CAD build for the part. Positions are in the model's coordinates, mm. Face numbers are marked on the shaded views. A direction names the side the tool comes from. Round coordinates to 2 decimals unless told otherwise and drop trailing zeros. Loops run counter-clockwise (first coordinate to the right, second up) from the corner with the lowest first, then second, coordinate; pieces in that order, holes last. Notation, with made-up numbers: M 25.5,88 L 35.5,88 A17 cw 35.5,92 Z; hole C -39,86.25 d1. An arc over 180 degrees is marked long. Use one line per item in the form item = value.
from build123d import *

# Parameters (mm, degrees)
F0_W        = 88.9
F0_H        = 38.1
F1_DEPTH    = 9.144
F2_R        = 4.572
F3_DEPTH    = 12.7
F4_R        = 9.525
F5_DEPTH    = 21.845
F6_SIZE     = 9.144
F7_W        = 9.144
F7_H        = 19.812
F8_DEPTH    = 50.8
F9_T1_DEPTH = 35.2722991577
F10_R       = 4.7625
F11_DEPTH   = 9.144


# Not quite as in the source:
# - a fillet or chamfer that OpenCascade refuses, or shapes differently, is made with other operations: its cross-section is extruded or revolved along the edge and cut away or added


with BuildPart() as f1:
    # F0 (on Front) → F1 (new body)
    with BuildSketch(Plane.XZ):
        with Locations((44.45, 19.05)):
            Rectangle(F0_W, F0_H)
    extrude(amount=F1_DEPTH)

    # F2 (on face) → F3 (join)
    with BuildSketch(Plane.XZ.offset(9.144)):
        with Locations((12.2043658048, 19.05)):
            Circle(F2_R)
    extrude(amount=F3_DEPTH)

    # F4 (on face) → F5 (cut, through all)
    with BuildSketch(Plane(origin=(0, 0, 0), x_dir=(-1, 0, 0), z_dir=(0, 1, 0))):
        with Locations((-76.2, 19.05)):
            Circle(F4_R)
    extrude(amount=-F5_DEPTH, mode=Mode.SUBTRACT)

    # F6
    f6_edges = [f1.edges().sort_by_distance(p)[0] for p in [
        (0, -4.572, 38.1),
        (88.9, -4.572, 38.1),
        (0, -4.572, 0),
        (88.9, -4.572, 0),
    ]]
    chamfer(f6_edges, length=F6_SIZE)

    # F7 (on face) → F8 (join)
    with BuildSketch(Plane.YZ.offset(88.9)):
        with Locations((-4.572, 19.05)):
            Rectangle(F7_W, F7_H)
    extrude(amount=F8_DEPTH)

    # F9: chamfer of 5.08 on 4 edges, made by hand

    # F9_s2 → F9_t1 (cut)
    with BuildSketch(Plane.XZ.offset(-13.0641495789)):
        Polygon((134.62, 28.956), (139.7, 23.876), (139.7, 28.956), align=None)
        Polygon((134.62, 9.144), (139.7, 14.224), (139.7, 9.144), align=None)
    extrude(amount=F9_T1_DEPTH, mode=Mode.SUBTRACT)

    # F10 (on face) → F11 (join)
    with BuildSketch(Plane.XZ.offset(9.144)):
        with Locations((130.556, 18.669)):
            Circle(F10_R)
    extrude(amount=F11_DEPTH)


solid = f1.part
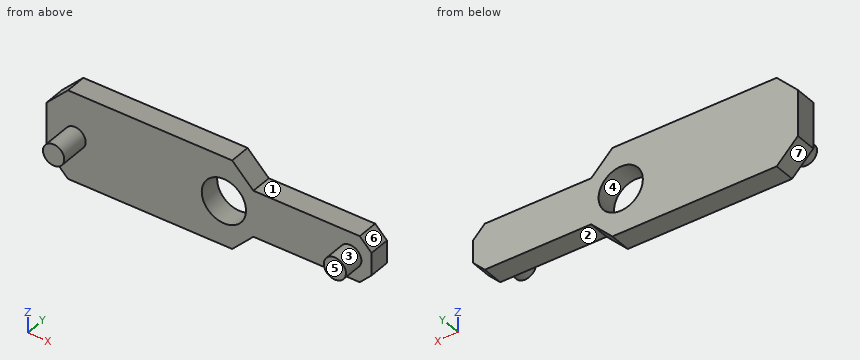
1. Cut at C-C on z = 11. Write the cut outline in (x, y), and give its area (3 significant figures).
Completed:
outline = M 0,-9.14 L 71.11,-9.14 L 71.11,0 L 0,0 Z; M 81.29,-9.14 L 136.48,-9.14 L 136.48,0 L 81.29,0 Z
area = 1,150 mm2
2. Cut at B-B on y = -1.25. Write the cut outline in (x, z) (3 decimals), and give its area (3 significant figures).
Completed:
outline = M 0,9.144 L 9.144,0 L 79.756,0 L 88.9,9.144 L 134.62,9.144 L 139.7,14.224 L 139.7,23.876 L 134.62,28.956 L 88.9,28.956 L 79.756,38.1 L 9.144,38.1 L 0,28.956 Z; hole C 76.2,19.05 d19.05
area = 3,920 mm2
3. Cut at D-D on x = 129. Write the cut outline in (y, z), and give its area (3 significant figures).
Completed:
outline = M -18.29,14.17 L -9.14,14.17 L -9.14,9.14 L 0,9.14 L 0,28.96 L -9.14,28.96 L -9.14,23.17 L -18.29,23.17 Z
area = 263 mm2
4. Probe line 1 along Z through (x, y) = (76.2, -3.75) (3 decimals); line 2 along X through (y, z) = (-2, 18.5); line 3 along Y through (x, z) = (54, 11). List the from-to ranges inside material, lowest first. Write a range as from..to.
Completed:
line_1 = 0..9.525, 28.575..38.1
line_2 = 0..66.69, 85.71..139.7
line_3 = -9.14..0
5. Tool access for the marked faces 1, 2 and 3: list every direction of +Z, -Z, +X, -X, +Y, -Y with a clear straight run to the whole face (end or side of a thin tool).
Completed:
face_1 = +Z, +X, +Y, -Y
face_2 = -Z, +X, +Y, -Y
face_3 = -Y
6. Drop flat-ended pins along their axis: P1, Ø10.5, axis at x = 128.5, z = 18.5, coming from the -Y side; P2, Ø8, axis at x = 24, z = 10, coming from the -Y side; P3, Ø1, axis at x = 79.5, y = -11.5, coming from the -Z side; P4, Ø2.5, axis at x = 102.5, y = -4, coming from the +Z side. Give the stop position or say it passes through.
Completed:
P1 = -18.29
P2 = -9.14
P3 = through
P4 = 28.96
7. Cut at A-A on x = 76.2. Write the cut outline in (y, z) (3 decimals), and give its area (3 significant figures).
Completed:
outline = M -9.144,0 L 0,0 L 0,9.525 L -9.144,9.525 Z; M -9.144,28.575 L 0,28.575 L 0,38.1 L -9.144,38.1 Z
area = 174 mm2
8. Pull direction X, two halves, no side cores. Call the marked faces 4, 5, 6 and 7: +X half, -X half, draft (parallel to the pull), parting line (faces both ways), or undercut.
Completed:
face_4 = undercut
face_5 = draft
face_6 = +X half
face_7 = -X half
